The listing builds one solid part. Answer for the finished solid, in the listing's coordinates (mm). Coordinates: 2 decimals unless noted, no trailing zeros. Order: outer loops, then holes, each group sorted by start corner. A loop starts at its lowest first (then second) coordinate and runs counter-clockwise, first axis right, second up.
from build123d import *

# Parameters (mm, degrees)
BOSS_EXTRUDE1_DEPTH = 3.175
CUT_EXTRUDE1_REACH  = 5.175
SKETCH2_R           = 2.75


with BuildPart() as part:
    # Sketch1 → Boss-Extrude1 (new body)
    with BuildSketch(Plane.XY):
        Polygon((0, 0), (20, 0), (20, 20), (40, 20), (40, -20), (0, -20), align=None)
    extrude(amount=BOSS_EXTRUDE1_DEPTH)

    # Sketch2 → Cut-Extrude1 (cut, up to next)
    with BuildSketch(Plane.XY.offset(3.175), mode=Mode.PRIVATE) as cut_extrude1_sk1:
        with Locations((30, 10)):
            Circle(SKETCH2_R)
    cut_extrude1_tool1 = extrude(cut_extrude1_sk1.sketch, amount=-CUT_EXTRUDE1_REACH, mode=Mode.PRIVATE) & part.part
    add(cut_extrude1_tool1.solids().sort_by_distance((30, 10, 3.175))[0], mode=Mode.SUBTRACT)


solid = part.part
1) This flat-tipped pin is pushed along its axis until it touches: P1, Ø1.6, axis at x = 13, z = 2.5, coming from the +Y side. Where does it stop, or does it pass through?
2) Section A-A (x = 30) is taken. Give the vertices of the cut face in (y, z) (3 decimals), then the cut area to 3 significant figures.
3) Section D-D (y = 5) is taken. Give the vertices of the cut face in (x, z) (3 decimals).
4) Determine the mould class of faces 1 (the face through (20, -20, 2)), 2 (the face through (20, 10, 2)), 3 (the face through (27.253, 10.121, 1.61)), 4 (the face through (10, 0, 2)) for opening direction Y: released by +Y, released by -Y, zero draft, split by the parting line, or undercut.
5) Consider L1, parallel to Y at x = 30, z = 1.9; L2, parallel to X at y = 14, z = 2.9; L3, parallel to X at y = 9.5, z = 0.45. Determine where each line is inside the solid, lowest interval first.
6) Section B-B (z = 2.5) is taken. Give the vertices of the cut face in (x, y), then the cut area to 3 significant figures.
7) Section C-C (y = 11) is taken. Give the vertices of the cut face in (x, z) (3 decimals).
Filled sheet:
1. P1: stops at y = 0
2. outline: (-20, 0) - (7.25, 0) - (7.25, 3.175) - (-20, 3.175) - close; (12.75, 0) - (20, 0) - (20, 3.175) - (12.75, 3.175) - close
2. area: 110 mm2
3. outline: (20, 0) - (40, 0) - (40, 3.175) - (20, 3.175) - close
4. face 1: released by -Y
4. face 2: zero draft
4. face 3: undercut
4. face 4: released by +Y
5. L1: y = -20 to 7.25, 12.75 to 20
5. L2: x = 20 to 40
5. L3: x = 20 to 27.3, 32.7 to 40
6. outline: (0, -20) - (40, -20) - (40, 20) - (20, 20) - (20, 0) - (0, 0) - close; hole circle Ø5.5 at (30, 10)
6. area: 1,180 mm2
7. outline: (20, 0) - (27.438, 0) - (27.438, 3.175) - (20, 3.175) - close; (32.562, 0) - (40, 0) - (40, 3.175) - (32.562, 3.175) - close
